Build history of the part. All positions in model axes, mm. A direction names the side the tool comes from. Round coordinates to 2 decimals unless told otherwise and drop trailing zeros. Write each loop counter-clockwise with the first axis right and the second up, starting at its lowest first coordinate (ties: lowest second). Pieces come first, ordered by that corner, then holes.
Item 1: Mould opens along X. For faces 1 (the flat face through (0.1, -0.4, -2.5)), 2 (the flat face through (-5, 6, 0)), 3 (the flat face through (9.26, 5, 0)) say: +X half, -X half, draft (parallel to the pull), parting line (faces both ways), or undercut.
Item 2: Band-saw the part on A-A, the plane y = 8. Write the cut outline in (x, z), then the cut area to 3 significant figures.
Item 3: Band-saw the part on D-D, the plane z = -2.1. Write the cut outline in (x, y).
Item 4: Band-saw the part on C-C, the plane z = 0. Write the cut outline in (x, y) (3 decimals), then the cut area to 3 significant figures.
Item 5: 3-axis set-ups, long thin cutter, end or side, ignore diameter. For faces 4 (the cylindrical face through (-0.714, -3.641, 0.031)), 5 (the flat face through (0, -4.3, 0)), 6 (the flat face through (5, 6, 0)): which of +Z, -Z, +X, -X, +Y, -Y reach the whole face in a straight line?
Item 6: Band-saw the part on B-B, the plane x = 0. Write the cut outline in (y, z) (3 decimals).
Item 7: Wall check: probe 1 along X at (y, z) = (3.25, 0.45); probe 2 along Y at (x, z) = (-3.25, 0.1); probe 3 along Y at (x, z) = (8, 0). Give the ranges that are in metal, low to high.
Item 8: Drop flat-ended pins along their axis: pin 1 Ø1.5 at (x, z) = (-1.5, -0.5) entering from +Y; pin 2 Ø1.5 at (x, z) = (1.5, 1) entering from -Y. Give the stop position or say it passes through.
```python
from build123d import *

# Parameters (mm, degrees)
BOSS_EXTRUDE1_DEPTH = 2.5
SKETCH2_R           = 0.715
BOSS_EXTRUDE2_DEPTH = 1.3


with BuildPart() as part:
    # Sketch1 → Boss-Extrude1 (new body, symmetric)
    with BuildSketch(Plane.XY):
        Polygon((-9.26, -3), (-9.26, 12.2), (-5, 12.2), (-5, 0), (5, 0), (5, 12.2), (9.26, 12.2), (9.26, -3), align=None)
    extrude(amount=BOSS_EXTRUDE1_DEPTH, both=True)

    # Sketch2 → Boss-Extrude2 (add)
    with BuildSketch(Plane.XZ.offset(3)):
        Circle(SKETCH2_R)
    extrude(amount=BOSS_EXTRUDE2_DEPTH)


solid = part.part
```
Results:
1. face 1: draft
1. face 2: undercut
1. face 3: +X half
2. outline: (-9.26, -2.5) - (-5, -2.5) - (-5, 2.5) - (-9.26, 2.5) - close; (5, -2.5) - (9.26, -2.5) - (9.26, 2.5) - (5, 2.5) - close
2. area: 42.6 mm2
3. outline: (-9.26, -3) - (9.26, -3) - (9.26, 12.2) - (5, 12.2) - (5, 0) - (-5, 0) - (-5, 12.2) - (-9.26, 12.2) - close
4. outline: (-9.26, -3) - (-0.715, -3) - (-0.715, -4.3) - (0.715, -4.3) - (0.715, -3) - (9.26, -3) - (9.26, 12.2) - (5, 12.2) - (5, 0) - (-5, 0) - (-5, 12.2) - (-9.26, 12.2) - close
4. area: 161 mm2
5. face 4: -Y
5. face 5: +Z, -Z, +X, -X, -Y
5. face 6: +Z, -Z, +Y
6. outline: (-4.3, -0.715) - (-3, -0.715) - (-3, -2.5) - (0, -2.5) - (0, 2.5) - (-3, 2.5) - (-3, 0.715) - (-4.3, 0.715) - close
7. probe 1: x = -9.26 to -5, 5 to 9.26
7. probe 2: y = -3 to 0
7. probe 3: y = -3 to 12.2
8. pin 1: stops at y = 0
8. pin 2: stops at y = -3
